The listing builds one solid part. Answer for the finished solid, in the listing's coordinates (mm). Face numbers are marked on the shaded views. A direction names the side the tool comes from. Coordinates: 2 decimals unless noted, no trailing zeros. Loops run counter-clockwise (first coordinate to the right, second up) from the corner with the lowest first, then second, coordinate; pieces in that order, holes last. Notation, with made-up numbers: (1, 7) - (34, 7) arc R31 ccw to (34, 45) - close; hole circle Ø3 at (21, 86.25). An arc over 180 degrees is marked (long way). Put each result on its own line as item: value.
```python
from build123d import *

# Parameters (mm, degrees)
F0_W     = 16
F0_H     = 3
F1_DEPTH = 22
F2_W     = 7.5
F2_H     = 3
F3_DEPTH = 6
F4_W     = 7.5
F4_H     = 3
F5_DEPTH = 6
F7_DEPTH = 3.001
F9_DEPTH = 28.001


with BuildPart() as f1:
    # F0 (on Front) → F1 (new body)
    with BuildSketch(Plane.XZ):
        Rectangle(F0_W, F0_H)
    extrude(amount=F1_DEPTH)

    # F2 (on face) → F3 (join)
    with BuildSketch(Plane.XZ.offset(22)):
        Rectangle(F2_W, F2_H)
    extrude(amount=F3_DEPTH)

    # F4 (on face) → F5 (join)
    with BuildSketch(Plane(origin=(0, 0, 0), x_dir=(-1, 0, 0), z_dir=(0, 1, 0))):
        Rectangle(F4_W, F4_H)
    extrude(amount=F5_DEPTH)

    # F6 (on face) → F7 (cut, through all)
    with BuildSketch(Plane.XY.offset(1.5)):
        Polygon((-8, -1.5746736809), (-8, -2.4259408148), (-7.574366433, -2.0003072478), align=None)
        Polygon((-8, -2.5746736809), (-8, -3.4259408148), (-7.574366433, -3.0003072478), align=None)
        Polygon((-8, -3.5746736809), (-8, -4.4259408148), (-7.574366433, -4.0003072478), align=None)
        Polygon((-8, -4.5746736809), (-8, -5.4259408148), (-7.574366433, -5.0003072478), align=None)
        Polygon((-8, -5.5746736809), (-8, -6.4259408148), (-7.574366433, -6.0003072478), align=None)
        Polygon((-8, -6.5746736809), (-8, -7.4259408148), (-7.574366433, -7.0003072478), align=None)
        Polygon((-8, -7.5746736809), (-8, -8.4259408148), (-7.574366433, -8.0003072478), align=None)
        Polygon((-8, -8.5746736809), (-8, -9.4259408148), (-7.574366433, -9.0003072478), align=None)
        Polygon((-8, -9.5746736808), (-8, -10.4259408148), (-7.574366433, -10.0003072478), align=None)
        Polygon((-7.574366433, -11.0003072478), (-8, -10.5746736808), (-8, -11.4259408148), align=None)
        Polygon((-7.566103496, -12.0002731092), (-8, -11.5663766052), (-8, -12.4341696131), align=None)
        Polygon((-7.557840559, -13.0002389705), (-8, -12.5580795295), (-8, -13.4423984115), align=None)
        Polygon((-7.549577622, -14.0002048319), (-8, -13.5497824539), (-8, -14.4506272099), align=None)
        Polygon((-7.541314685, -15.0001706932), (-8, -14.5414853782), (-8, -15.4588560082), align=None)
        Polygon((-7.5, -20), (-8, -19.5), (-8, -20.5), align=None)
        Polygon((-7.508262937, -19.0000341386), (-8, -18.5082970756), (-8, -19.4917712016), align=None)
        Polygon((-7.516525874, -18.0000682773), (-8, -17.5165941513), (-8, -18.4835424033), align=None)
        Polygon((-7.524788811, -17.0001024159), (-8, -16.5248912269), (-8, -17.4753136049), align=None)
        Polygon((-7.533051748, -16.0001365546), (-8, -15.5331883026), (-8, -16.4670848066), align=None)
    extrude(amount=-F7_DEPTH, mode=Mode.SUBTRACT)

    # F8 (on face) → F9 (cut, through all)
    with BuildSketch(Plane.XZ.offset(22)):
        Polygon((-7.4629583396, -1.5), (-8, 1.5), (-8, -1.5), align=None)
    extrude(amount=-F9_DEPTH, mode=Mode.SUBTRACT)


solid = f1.part
```
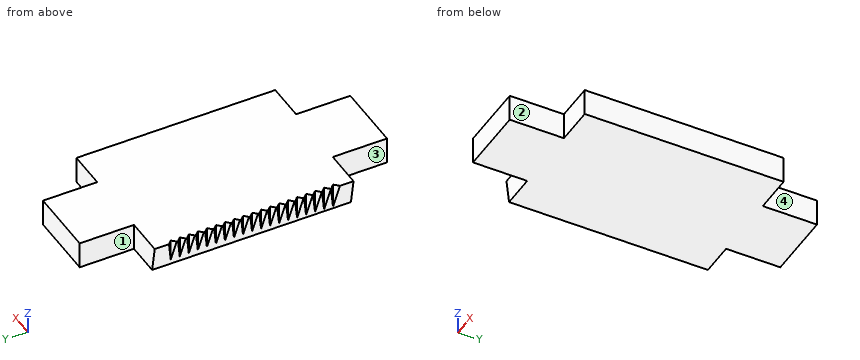
1) For the marked faces 1, 2, 3 and 4, determine the directions among +Z, -Z, +X, -X, +Y, -Y from which every point of the face is accessible in a straight line to the end or side of a thin tool.
Found:
face 1: +Z, -Z, -X, +Y
face 2: +Z, -Z, +X, -Y
face 3: +Z, -Z, -X, -Y
face 4: +Z, -Z, +X, +Y
2) Straight lines are drawn through the part: L1, parallel to Y at x = 4.75, z = 0.15; L2, parallel to X at y = 3.5, z = -1.05; L3, parallel to X at y = -9, z = -1. For each, find the intervals that lie inside material, in ascending order. Write a range as [from, to].
Found:
L1: y = [-22, 0]
L2: x = [-3.75, 3.75]
L3: x = [-7.55, 8]
3) Each of these flat-tipped pins is pushed along its axis until it touches: pin 1 (0.9 mm diameter, centred on x = 7, z = 0.5, fed in from -Y); pin 2 (0.9 mm diameter, centred on y = -26.5, z = -0.5, fed in from +X); pin 3 (1.5 mm diameter, centred on y = -26, z = 0.5, fed in from -X). Where does it stop, or does it pass through?
Found:
pin 1: stops at y = -22
pin 2: stops at x = 3.75
pin 3: stops at x = -3.75
4) The part is cut by section A-A (y = -22.5). Give the vertices of the cut face in (x, z).
Found:
outline: (-3.75, -1.5) - (3.75, -1.5) - (3.75, 1.5) - (-3.75, 1.5) - close
5) The part is cut by section B-B (x = 5). Give the vertices of the cut face in (y, z).
Found:
outline: (-22, -1.5) - (0, -1.5) - (0, 1.5) - (-22, 1.5) - close
